For this review, use the dimensioned drawing (mm, ordinates from the lowest corner) and the shaded views. A direction names the side the tool comes from. Coordinates: 2 decimals unless noted, no trailing zeros. Loops run counter-clockwise (first coordinate to the right, second up) from the corner with the lowest first, then second, coordinate; pieces in that order, holes last. Notation, with made-up numbers: (67.25, 20.25) -> (111.25, 20.25) arc R19 ccw to (111.25, 57.25) -> close; hole circle Ø5 at (30, 52.5). An arc over 180 degrees is marked (long way). Use one line per item in the form item = value. Start each with the question number.
1. Consider section D-D (z = 6). State the section outline as (x, y) points.
2. Consider section B-B (z = 62.5). State the section outline as (x, y) points, then the cut area to 3 significant figures.
3. The part is to be moulded in two halves that separate along X. For the marked faces 1, 2, 3 and 4, say which applies: released by +X, released by -X, zero draft, split by the parting line, or undercut.
4. Wall thickness on line 1 (X direction, y = 27.5, z = 54.5); line 2 (X direction, y = 60, z = 51.5); line 3 (Y direction, x = 64, z = 35): over which ranges is each line inside the solid? List them lowest first. Write a range as from..to.
5. Consider section C-C (y = 61). State the section outline as (x, z) points, then the cut area to 4 significant figures.
6. For pin 1 (10.5 mm diameter, centred on x = 85, z = 25, fed in from -Y); pin 2 (1.5 mm diameter, centred on y = 33, z = 29.5, fed in from -X); pin 3 (3 mm diameter, centred on x = 71, y = 57, fed in from +Z); pin 4 (15 mm diameter, centred on x = 54.5, z = 29.5, fed in from -Y), all flat-tipped, find the tip position at first contact; note any pin that passes through.
7. Consider section A-A (y = 26). State the section outline as (x, z) points.
8. Machinability: for the marked faces 5, 6 and 7, which of the approach directions +Z, -Z, +X, -X, +Y, -Y give a long, thin tool a straight path to every point of the face, cutting with its end or side? Answer none if there is none.
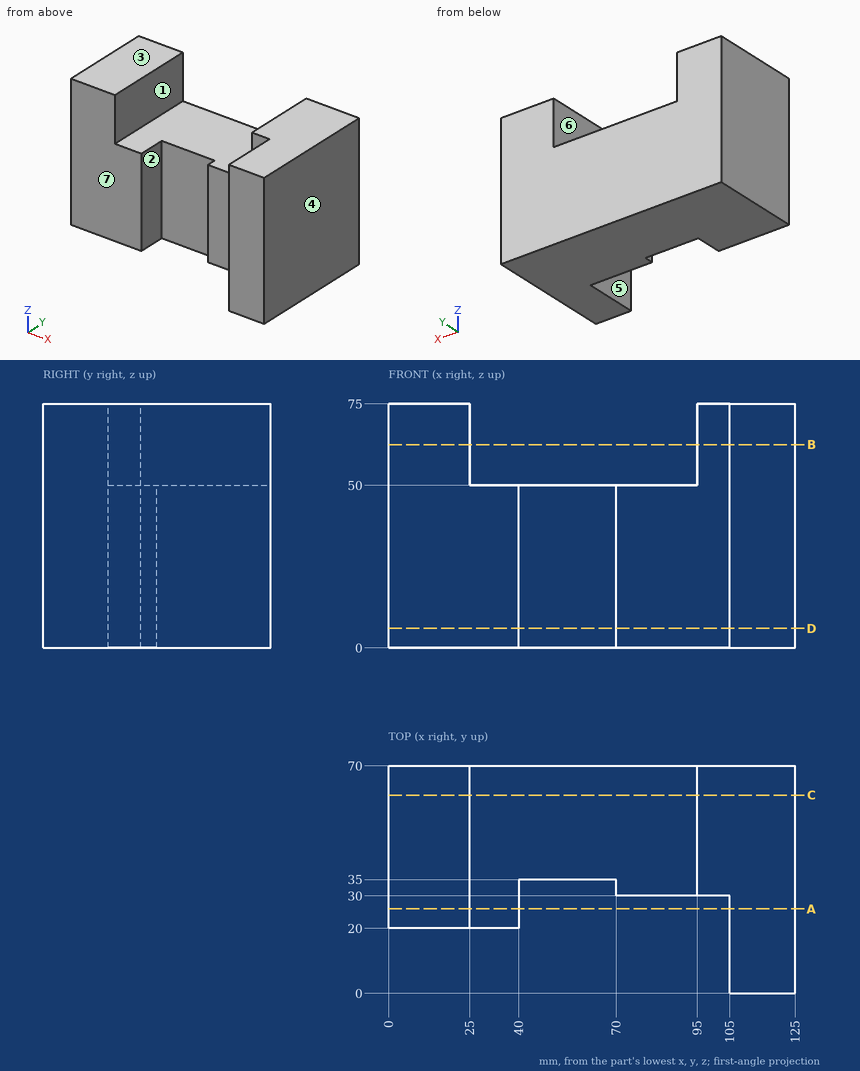
Geometry check:
q1.outline = (0, 20) -> (40, 20) -> (40, 35) -> (70, 35) -> (70, 30) -> (105, 30) -> (105, 0) -> (125, 0) -> (125, 70) -> (0, 70) -> close
q2.outline = (0, 20) -> (25, 20) -> (25, 70) -> (0, 70) -> close; (95, 30) -> (105, 30) -> (105, 0) -> (125, 0) -> (125, 70) -> (95, 70) -> close
q2.area = 3,050 mm²
q3.face_1 = undercut
q3.face_2 = undercut
q3.face_3 = zero draft
q3.face_4 = released by +X
q4.line_1 = 0..25, 105..125
q4.line_2 = 0..25, 95..125
q4.line_3 = 35..70
q5.outline = (0, 0) -> (125, 0) -> (125, 75) -> (95, 75) -> (95, 50) -> (25, 50) -> (25, 75) -> (0, 75) -> close
q5.area = 7,625 mm²
q6.pin_1 = 30
q6.pin_2 = 0
q6.pin_3 = 50
q6.pin_4 = 35
q7.outline = (0, 0) -> (40, 0) -> (40, 50) -> (25, 50) -> (25, 75) -> (0, 75) -> close; (105, 0) -> (125, 0) -> (125, 75) -> (105, 75) -> close
q8.face_5 = +Z, -Z, -Y
q8.face_6 = +Z, +Y, -Y
q8.face_7 = +Z, -Z, -X, -Y
